```python
from build123d import *

# Parameters (mm, degrees)
F0_W     = 41
F0_H     = 41
F0_W_2   = 10
F0_H_2   = 10
F1_DEPTH = 10
F2_DEPTH = 25
F3_R     = 10
F4_DEPTH = 8
F6_DEPTH = 25
F7_DEPTH = 1.5
F8_DEPTH = 10
F9_DEPTH = 3


# Not quite as in the source:
# - a fillet or chamfer that OpenCascade refuses, or shapes differently, is made with other operations: its cross-section is extruded or revolved along the edge and cut away or added


with BuildPart() as f1:
    # F0 (on Top) → F1 (new body)
    with BuildSketch(Plane.XY):
        Rectangle(F0_W, F0_H)
        Rectangle(F0_W_2, F0_H_2, mode=Mode.SUBTRACT)
        Rectangle(F0_W_2, F0_H_2)
    extrude(amount=F1_DEPTH)

    # F0 (on Top) → F2 (join)
    with BuildSketch(Plane.XY):
        Rectangle(F0_W_2, F0_H_2)
    extrude(amount=F2_DEPTH)

    # F3 (on face) → F4 (join)
    with BuildSketch(Plane.XY.offset(25)):
        Circle(F3_R)
    extrude(amount=-F4_DEPTH)

    # F5 (on face) → F6 (cut)
    with BuildSketch(Plane(origin=(0, 0, 0), x_dir=(1, 0, 0), z_dir=(0, 0, -1))):
        with BuildLine():
            Line((0, 20.5), (0, 16.625))
            ThreePointArc((0, 16.625), (14.2014511666, 13.1849661001), (20.5, 0))
            Line((20.5, 0), (20.5, 20.5))
            Line((20.5, 20.5), (0, 20.5))
        make_face()
        with BuildLine():
            Line((20.5, -20.5), (20.5, 0))
            Line((20.5, 0), (16.625, 0))
            ThreePointArc((16.625, 0), (13.15340166, -14.1758531755), (0, -20.5))
            Line((0, -20.5), (20.5, -20.5))
        make_face()
        with BuildLine():
            ThreePointArc((0, -16.625), (-14.1919455674, -13.1732449101), (-20.5, 0))
            Line((-20.5, 0), (-20.5, -20.5))
            Line((-20.5, -20.5), (0, -20.5))
            Line((0, -20.5), (0, -16.625))
        make_face()
        with BuildLine():
            ThreePointArc((-16.625, 0), (-13.1636820987, 14.1841903605), (0, 20.5))
            Line((0, 20.5), (-20.5, 20.5))
            Line((-20.5, 20.5), (-20.5, 0))
            Line((-20.5, 0), (-16.625, 0))
        make_face()
    extrude(amount=-F6_DEPTH, mode=Mode.SUBTRACT)

    # F7 (cut): a face of the model
    f7_faces = [f1.faces().sort_by_distance(p)[0] for p in [
        (0, 0, 25),
    ]]
    extrude(f7_faces, amount=-F7_DEPTH, mode=Mode.SUBTRACT)

    # F8 (cut): a face of the model
    f8_faces = [f1.faces().sort_by_distance(p)[0] for p in [
        (0.0007164835, -0.0062799282, 0),
    ]]
    extrude(f8_faces, amount=-F8_DEPTH, mode=Mode.SUBTRACT)

    # F9 (add): a face of the model
    f9_faces = [f1.faces().sort_by_distance(p)[0] for p in [
        (-9.7171572875, 0, 17),
    ]]
    extrude(f9_faces, amount=F9_DEPTH)

    # F10: chamfer of 5 on 1 edges, made by hand


with BuildPart() as f10_tool2:
    # F10_s3 → F10_t4 (revolve)
    with BuildSketch(Plane.XZ):
        Polygon((5, 14), (10, 19), (10, 14), align=None)
    revolve(axis=Axis((0, 0, 14), (0, 0, 1)))

    split(bisect_by=Plane.YZ.offset(5), keep=Keep.TOP)


with BuildPart() as f1_1:
    add(f1.part)

    # F10_t1: cut F10_tool2
    add(f10_tool2.part, mode=Mode.SUBTRACT)


with BuildPart() as f10_tool7:
    # F10_s8 → F10_t9 (revolve)
    with BuildSketch(Plane.XZ):
        Polygon((5, 14), (10, 19), (10, 14), align=None)
    revolve(axis=Axis((0, 0, 14), (0, 0, 1)))

    split(bisect_by=Plane.XZ.offset(-5), keep=Keep.BOTTOM)


with BuildPart() as f1_2:
    add(f1_1.part)

    # F10_t6: cut F10_tool7
    add(f10_tool7.part, mode=Mode.SUBTRACT)


with BuildPart() as f10_tool12:
    # F10_s13 → F10_t14 (revolve)
    with BuildSketch(Plane.XZ):
        Polygon((5, 14), (10, 19), (10, 14), align=None)
    revolve(axis=Axis((0, 0, 14), (0, 0, 1)))

    split(bisect_by=Plane.YZ.offset(-5), keep=Keep.BOTTOM)


with BuildPart() as f1_3:
    add(f1_2.part)

    # F10_t11: cut F10_tool12
    add(f10_tool12.part, mode=Mode.SUBTRACT)


with BuildPart() as f10_tool17:
    # F10_s18 → F10_t19 (revolve)
    with BuildSketch(Plane.XZ):
        Polygon((5, 14), (10, 19), (10, 14), align=None)
    revolve(axis=Axis((0, 0, 14), (0, 0, 1)))

    split(bisect_by=Plane.XZ.offset(5), keep=Keep.TOP)


with BuildPart() as f1_4:
    add(f1_3.part)

    # F10_t16: cut F10_tool17
    add(f10_tool17.part, mode=Mode.SUBTRACT)


solid = f1_4.part
```
Model file for the job. Use its own axes, mm. Coordinates: 2 decimals unless noted, no trailing zeros. Write each loop counter-clockwise with the first axis right and the second up, starting at its lowest first coordinate (ties: lowest second). Pieces come first, ordered by that corner, then holes. Notation, with made-up numbers: (-21, 31) - (-1, 31) arc R18 ccw to (-1, 61) - close; hole circle Ø11 at (-25, -16.75). An arc over 180 degrees is marked (long way). One line per question, with ' | ' between items. Start each with the question number.
Q1. Cut at C-C, the plane z = 13.5. List the corners of the cut face in (x, y), then the cut area to 3 significant figures.
Q2. Pin check, flat tips, straight feed: pin 1 (2 mm diameter, centred on y = 4, z = 13, fed in from +X); pin 2 (3 mm diameter, centred on y = 1, z = 12.5, fed in from -X); pin 3 (3 mm diameter, centred on x = -2, z = 14.5, fed in from +Y). Stop position of each tip, or through.
Q3. Drill centre lines: line 1 (X direction, y = -4.75, z = 13); line 2 (Y direction, x = 0, z = 20.5). Where is each one in solid material? Low to high. Write a range as [from, to].
Q4. Cut at D-D, the plane z = 22. List the corners of the cut face in (x, y).
Q5. Cut at A-A, the plane x = 0. List the corners of the cut face in (y, z), then the cut area to 3 significant figures.
Answer below:
1) outline: (-5, -5) - (5, -5) - (5, 5) - (-5, 5) - close | area: 100 mm^2
2) pin 1: x = 5 | pin 2: x = -5 | pin 3: y = 6.76
3) line 1: [-5, 5] | line 2: [-10, 10]
4) outline: circle Ø20 at (0, 0)
5) outline: (-10, 19) - (-5, 14) - (-5, 10) - (5, 10) - (5, 14) - (10, 19) - (10, 23.5) - (-10, 23.5) - close | area: 205 mm^2
